CAD build for the part. Positions are in the model's coordinates, mm. A direction names the side the tool comes from. Coordinates: 2 decimals unless noted, no trailing zeros. Loops run counter-clockwise (first coordinate to the right, second up) from the corner with the lowest first, then second, coordinate; pieces in that order, holes last. Notation, with made-up numbers: (-18, 15.25) - (11, 15.25) arc R19 cw to (11, 31.25) - close; hole circle Ø5 at (-23, 35). An arc over 180 degrees is marked (long way). Put each result on its own line as item: value.
```python
from build123d import *

# Parameters (mm, degrees)
SKETCH2_R           = 1
BOSS_EXTRUDE1_DEPTH = 1
FILLET1_R           = 1.861618014
FILLET2_R           = 0.465404504


with BuildPart() as part:
    # Sketch2 → Boss-Extrude1 (new body, symmetric)
    with BuildSketch(Plane.XY):
        with BuildLine():
            Line((-8.762233136, -15.726474067), (-8.096527006, -10.551599426))
            ThreePointArc((-8.096527006, -10.551599426), (-13.401846727, 5.188067163), (0, 15))
            Line((0, 15), (0, 11.6))
            ThreePointArc((0, 11.6), (-11.599558308, 0.101227812), (-0.202447915, -11.598233264))
            Line((-0.202447915, -11.598233264), (-0.314191169, -18))
            ThreePointArc((-0.314191169, -18), (-4.678418491, -17.384220331), (-8.762233136, -15.726474067))
        make_face()
        with Locations((-3.84647005, -14.292839124)):
            Circle(SKETCH2_R, mode=Mode.SUBTRACT)
    extrude(amount=BOSS_EXTRUDE1_DEPTH, both=True)

    # Fillet1
    fillet1_edges = [part.edges().sort_by_distance(p)[0] for p in [
        (-8.096527006, -10.551599426, 0),
    ]]
    fillet(fillet1_edges, radius=FILLET1_R)

    # Fillet2
    fillet2_edges = [part.edges().sort_by_distance(p)[0] for p in [
        (-8.762233136, -15.726474067, 0),
    ]]
    fillet(fillet2_edges, radius=FILLET2_R)

    # Mirror1: part across face


with BuildPart() as part_1:
    add(part.part)
    add(part.part.mirror(Plane(origin=(0, 13.3, 0), x_dir=(0, 0, 1), z_dir=(1, 0, 0))))


solid = part_1.part
```
Q1. Slice it at A-A, the plane y = 8. Give the cut face in (x, z), then the cut area to 3 significant figures.
Determined:
outline: (-12.16, -1) - (-8.4, -1) - (-8.4, 1) - (-12.16, 1) - close; (8.4, -1) - (12.16, -1) - (12.16, 1) - (8.4, 1) - close
area: 15.0 mm2
Q2. Wall check: L1, parallel to Y at x = -3.75, z = -0.25; L2, parallel to Y at x = 3, z = -0.2; L3, parallel to Y at x = 9.25, z = 0.8. Give the ranges that are in metal, low to high. Write a range as from..to.
Determined:
L1: -17.61..-15.29, -13.3..-10.98, 10.98..14.49
L2: -17.75..-14.83, -13.76..-11.21, 11.21..14.68
L3: -9.65..-7, 7..11.53
Q3. Pin check, flat tips, straight feed: pin 1 Ø3 at (x, y) = (-3.85, -14.29) entering from +Z; pin 2 Ø1 at (y, z) = (-1.5, 0.5) entering from +X; pin 3 Ø1 at (x, z) = (6.5, -0.5) entering from -Y. Stop position of each tip, or through.
Determined:
pin 1: z = 1
pin 2: x = 13.92
pin 3: y = -16.97
Q4. Slice it at B-B, the plane x = -5.5. Give the cut face in (y, z).
Determined:
outline: (-17.14, -1) - (-10.21, -1) - (-10.21, 1) - (-17.14, 1) - close; (10.21, -1) - (13.88, -1) - (13.88, 1) - (10.21, 1) - close
Q5. Slice it at C-C, the plane x = 3.25. Give the cut face in (y, z).
Determined:
outline: (-17.71, -1) - (-15.1, -1) - (-15.1, 1) - (-17.71, 1) - close; (-13.49, -1) - (-11.14, -1) - (-11.14, 1) - (-13.49, 1) - close; (11.14, -1) - (14.62, -1) - (14.62, 1) - (11.14, 1) - close
Q6. Slice it at D-D, the plane z = 0.35. Give the cut face in (x, y).
Determined:
outline: (-8.9, -9.94) arc R1.86 cw to (-8.23, -11.62) - (-8.72, -15.41) arc R0.47 ccw to (-8.48, -15.88) arc R18 ccw to (-0.31, -18) - (-0.2, -11.6) arc R11.6 cw (long way) to (0.2, -11.6) - (0.31, -18) arc R18 ccw to (8.48, -15.88) arc R0.47 ccw to (8.72, -15.41) - (8.23, -11.62) arc R1.86 cw to (8.9, -9.94) arc R14.06 ccw (long way) to start; hole circle Ø2 at (-3.85, -14.29); hole circle Ø2 at (3.85, -14.29)
Q7. Mould opens along Y. For faces 1 (the cylindrical face through (-8.346, -10.705, -0.014)), 2 (the cylindrical face through (4.46, -17.44, 0.01)), 3 (the flat face through (-4.2, -11.2, -1)), 4 (the cylindrical face through (-4.846, -14.249, -0.014)) say: +Y half, -Y half, draft (parallel to the pull), parting line (faces both ways), or undercut.
Determined:
face 1: undercut
face 2: -Y half
face 3: draft
face 4: undercut
Q8. Tool access for faces 5 (the flat face through (8.48, -13.54, 0.01)), 6 (the flat face through (-8.48, -13.54, 0.01)), 7 (the flat face through (-4.2, -11.2, 1)): list every direction of +Z, -Z, +X, -X, +Y, -Y with a clear straight run to the whole face (end or side of a thin tool).
Determined:
face 5: +Z, -Z, +X
face 6: +Z, -Z, -X
face 7: +Z, +X, -X, +Y, -Y
